Can you work these out from the model? Positions are in its coordinate system, mm. Coordinates: 2 decimals unless noted, no trailing zeros. Loops run counter-clockwise (first coordinate to the right, second up) from the corner with the lowest first, then second, coordinate; pieces in that order, holes last. Notation, with made-up numbers: (71, 25.5) -> (104, 25.5) arc R12 ccw to (104, 31.5) -> close; hole circle Ø3 at (5.5, -25). An arc over 180 degrees is marked (long way). Use one line per item in the form item = value. Start each with the question number.
(1) Imagine slicing it at A-A (z = 2.35). List the corners of the cut face in (x, y) for me.
(2) I'm going to push flat-ended pins straight in: pin 1 (1 mm diameter, centred on y = 7, z = 3.5, fed in from +X); pin 2 (1 mm diameter, centred on y = -3.5, z = 2, fed in from -X). Where does each tip first touch, or does it pass through?
(3) Imagine slicing it at C-C (x = 50). List the corners of the cut face in (y, z) for me.
(4) Imagine slicing it at B-B (x = 87.5). List the corners of the cut face in (y, z) for me, plus the area to 3 significant figures.
(5) I need wall thicknesses on line 1 (Y direction, x = 87.5, z = 2.85); line 2 (Y direction, x = 160, z = 3.1); line 3 (X direction, y = 2.25, z = 3.6). Which ranges of each line are inside material? Lowest first, please. Write a range as [from, to].
(6) Thinking about a two-plate mould opening in Y: for faces 1 (the flat face through (79, 9, 2)), 2 (the cylindrical face through (46, 0, 2)), 3 (the flat face through (81, 0, 0)), which applies, released by +Y, released by -Y, zero draft, split by the parting line, or undercut?
```python
from build123d import *

# Parameters (mm, degrees)
SKETCH_1_R          = 1.25
SKETCH_1_R_2        = 3
SKETCH_1_R_3        = 4
EXTRUDE_1_DEPTH     = 4
SKETCH_2_R          = 1.5
CUT_EXTRUDE_1_DEPTH = 170.286738996


with BuildPart() as part:
    # ｽｹｯﾁ1 → ﾎﾞｽ - 押し出し1 (new body)
    with BuildSketch(Plane.XY):
        with BuildLine():
            Line((0, 9), (160, 9))
            ThreePointArc((160, 9), (169, 0), (160, -9))
            Line((160, -9), (0, -9))
            ThreePointArc((0, -9), (-9, 0), (0, 9))
        make_face()
        with Locations((160, 0)):
            Circle(SKETCH_1_R, mode=Mode.SUBTRACT)
        with Locations((100, 0)):
            Circle(SKETCH_1_R_2, mode=Mode.SUBTRACT)
        with Locations((50, 0)):
            Circle(SKETCH_1_R_3, mode=Mode.SUBTRACT)
    extrude(amount=EXTRUDE_1_DEPTH)

    # ｽｹｯﾁ2 → ｶｯﾄ - 押し出し1 (cut, through all)
    with BuildSketch(Plane.XY.offset(4)):
        with Locations((112.5, 0)):
            Circle(SKETCH_2_R)
        with Locations(Location((87.5, 0, 0), (0, 0, 180))):
            Circle(SKETCH_2_R)
    extrude(amount=-CUT_EXTRUDE_1_DEPTH, mode=Mode.SUBTRACT)


solid = part.part
```
Worked out:
q1.outline = (0, -9) -> (160, -9) arc R9 ccw to (160, 9) -> (0, 9) arc R9 ccw to start; hole circle Ø8 at (50, 0); hole circle Ø3 at (87.5, 0); hole circle Ø6 at (100, 0); hole circle Ø3 at (112.5, 0); hole circle Ø2.5 at (160, 0)
q2.pin_1 = 166.22
q2.pin_2 = -8.49
q3.outline = (-9, 0) -> (-4, 0) -> (-4, 4) -> (-9, 4) -> close; (4, 0) -> (9, 0) -> (9, 4) -> (4, 4) -> close
q4.outline = (-9, 0) -> (-1.5, 0) -> (-1.5, 4) -> (-9, 4) -> close; (1.5, 0) -> (9, 0) -> (9, 4) -> (1.5, 4) -> close
q4.area = 60.0 mm2
q5.line_1 = [-9, -1.5], [1.5, 9]
q5.line_2 = [-9, -1.25], [1.25, 9]
q5.line_3 = [-8.71, 46.69], [53.31, 98.02], [101.98, 168.71]
q6.face_1 = released by +Y
q6.face_2 = undercut
q6.face_3 = zero draft
